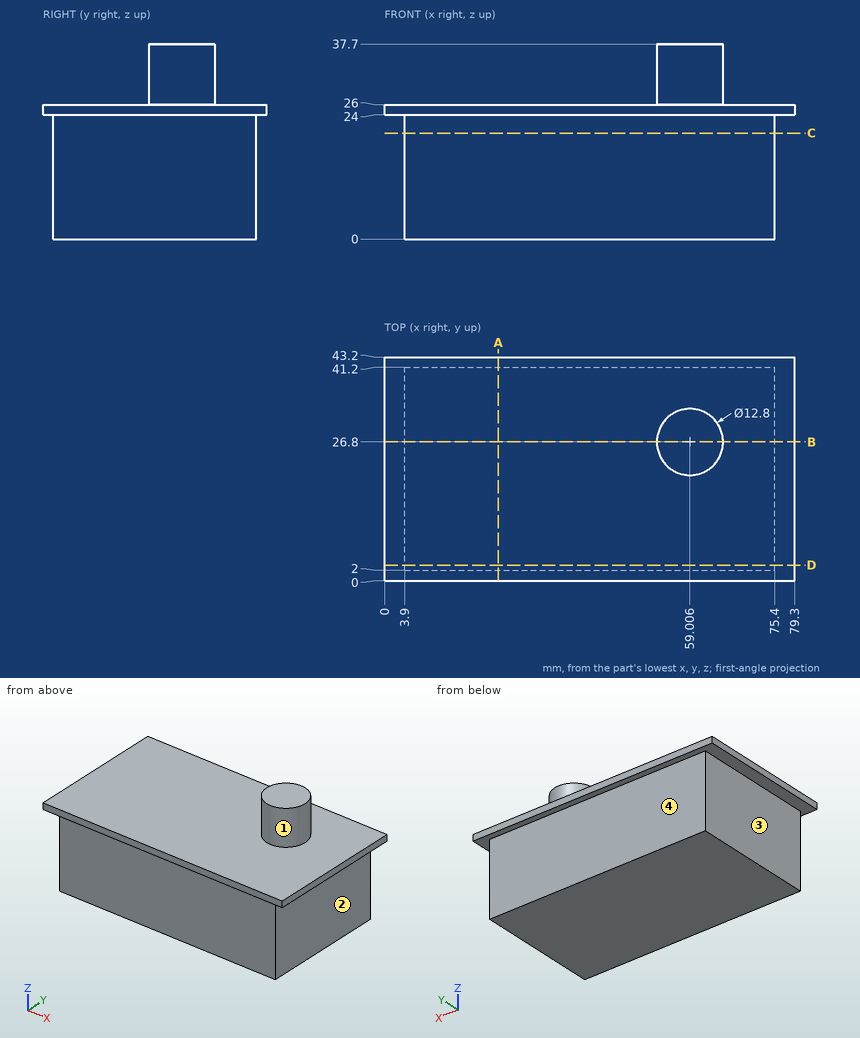
Geometry check sheet. Reference: drawing and pictorial views, mm from the part's lowest x, y, z. A direction names the side the tool comes from. Give positions to 0.01 mm unless a question says otherwise; leave off trailing zeros. Loops run counter-clockwise (first coordinate to the right, second up) from the corner with the lowest first, then second, coordinate; pieces in that order, holes last. Notation, with made-up numbers: M 65,80 L 113,80 A12 ccw 113,91 Z; hole C 32,-18.75 d10. An arc over 180 degrees is marked long. Use a Markdown table: item, result. Add a question column.
Q1. Sectioned sample at A-A, the plane x = 22. Record the cut outline in (y, z).
Q2. Scan lines: line 1 along Z through (x, y) = (17.5, 4); line 2 along Y through (x, z) = (15, 19); line 3 along X through (y, z) = (32.5, 23.5). Record each from-to range of solid material in increasing order. Write a range as [from, to].
Q3. Sectioned sample at D-D, the plane y = 3. Record the cut outline in (x, z).
Q4. Go/stop test with flat-tipped pins: pin 1 (19 mm diameter, centred on x = 32, z = 13.5, fed in from -Y); pin 2 (12 mm diameter, centred on x = 43.5, z = 8.5, fed in from +Y); pin 3 (10 mm diameter, centred on y = 38, z = 7.5, fed in from +X). Record where each tip stops, or that it passes through.
Q5. Sectioned sample at B-B, the plane y = 26.8. Record the cut outline in (x, z).
Q6. Sectioned sample at C-C, the plane z = 20.5. Record the cut outline in (x, y), then the cut area to 3 significant figures.
Q7. Tool access check on the marked faces 1, 2, 3 and 4. Record the directions out of +Z, -Z, +X, -X, +Y, -Y that give a thin tool (end or side, any length) a straight path to the whole face; none if there is none.
Verdict:
| question | item | result |
|---|---|---|
| 1 | outline | M 0,24 L 2,24 L 2,0 L 41.2,0 L 41.2,24 L 43.2,24 L 43.2,26 L 0,26 Z |
| 2 | line 1 | [0, 26] |
| 2 | line 2 | [2, 41.2] |
| 2 | line 3 | [3.9, 75.4] |
| 3 | outline | M 0,24 L 3.9,24 L 3.9,0 L 75.4,0 L 75.4,24 L 79.3,24 L 79.3,26 L 0,26 Z |
| 4 | pin 1 | y = 2 |
| 4 | pin 2 | y = 41.2 |
| 4 | pin 3 | x = 75.4 |
| 5 | outline | M 0,24 L 3.9,24 L 3.9,0 L 75.4,0 L 75.4,24 L 79.3,24 L 79.3,26 L 65.41,26 L 65.41,37.7 L 52.61,37.7 L 52.61,26 L 0,26 Z |
| 6 | outline | M 3.9,2 L 75.4,2 L 75.4,41.2 L 3.9,41.2 Z |
| 6 | area | 2,800 mm^2 |
| 7 | face 1 | +Z |
| 7 | face 2 | -Z, +X, +Y, -Y |
| 7 | face 3 | -Z, -X, +Y, -Y |
| 7 | face 4 | -Z, +X, -X, +Y |
